from build123d import *

# Parameters (mm, degrees)
BOSS_EXTRUDE1_DEPTH = 55
BOSS_EXTRUDE2_DEPTH = 4
CUT_EXTRUDE1_DEPTH  = 4
SKETCH6_R           = 7
BOSS_EXTRUDE3_DEPTH = 2
SKETCH7_R           = 6
CUT_EXTRUDE2_DEPTH  = 2
SKETCH8_R           = 1.613905717
CUT_EXTRUDE4_DEPTH  = 13
SKETCH9_R           = 6
CUT_EXTRUDE5_DEPTH  = 2
SKETCH11_R          = 1.615
CUT_EXTRUDE6_DEPTH  = 6
FILLET1_R           = 2
SKETCH14_R          = 7
SKETCH14_R_2        = 6
BOSS_EXTRUDE5_DEPTH = 2
CUT_EXTRUDE7_START  = -6
SKETCH15_R          = 1.615
SKETCH15_R_2        = 1.613905717
CUT_EXTRUDE7_DEPTH  = 6
SKETCH16_R          = 1
CUT_EXTRUDE9_DEPTH  = 6
CUT_EXTRUDE10_START = -6
SKETCH17_R          = 1
CUT_EXTRUDE10_DEPTH = 6
SKETCH18_W          = 2.103885612
SKETCH18_H          = 10
CUT_EXTRUDE12_DEPTH = 3
CUT_EXTRUDE13_REACH = 90.057
SKETCH19_R          = 0.8


with BuildPart() as part:
    # Sketch1 → Boss-Extrude1 (new body)
    with BuildSketch(Plane(origin=(0, 0, 0), x_dir=(1, 0, 0), z_dir=(0, 1, 0))):
        with BuildLine():
            Line((-43, 25), (43, 25))
            ThreePointArc((43, 25), (44.414213562, 24.414213562), (45, 23))
            Line((45, 23), (45, -23))
            ThreePointArc((45, -23), (44.414213562, -24.414213562), (43, -25))
            Line((43, -25), (-43, -25))
            ThreePointArc((-43, -25), (-44.414213562, -24.414213562), (-45, -23))
            Line((-45, -23), (-45, 23))
            ThreePointArc((-45, 23), (-44.414213562, 24.414213562), (-43, 25))
        make_face()
        with BuildLine():
            Line((-5, 18), (-5, -18))
            ThreePointArc((-5, -18), (-5.878679656, -20.121320344), (-8, -21))
            Line((-8, -21), (-39, -21))
            ThreePointArc((-39, -21), (-40.414213562, -20.414213562), (-41, -19))
            Line((-41, -19), (-41, 19))
            ThreePointArc((-41, 19), (-40.414213562, 20.414213562), (-39, 21))
            Line((-39, 21), (-8, 21))
            ThreePointArc((-8, 21), (-5.878679656, 20.121320344), (-5, 18))
        make_face(mode=Mode.SUBTRACT)
        with BuildLine():
            Line((41, 19), (41, -18))
            ThreePointArc((41, -18), (40.121320344, -20.121320344), (38, -21))
            Line((38, -21), (8, -21))
            ThreePointArc((8, -21), (5.878679656, -20.121320344), (5, -18))
            Line((5, -18), (5, 18))
            ThreePointArc((5, 18), (5.878679656, 20.121320344), (8, 21))
            Line((8, 21), (39, 21))
            ThreePointArc((39, 21), (40.414213562, 20.414213562), (41, 19))
        make_face(mode=Mode.SUBTRACT)
    extrude(amount=BOSS_EXTRUDE1_DEPTH)

    # Sketch2 → Boss-Extrude2 (add)
    with BuildSketch(Plane.XZ):
        with BuildLine():
            Line((45, 23), (45, -23))
            ThreePointArc((45, -23), (44.414213562, -24.414213562), (43, -25))
            Line((43, -25), (-43, -25))
            ThreePointArc((-43, -25), (-44.414213562, -24.414213562), (-45, -23))
            Line((-45, -23), (-45, 23))
            ThreePointArc((-45, 23), (-44.414213562, 24.414213562), (-43, 25))
            Line((-43, 25), (43, 25))
            ThreePointArc((43, 25), (44.414213562, 24.414213562), (45, 23))
        make_face()
    extrude(amount=-BOSS_EXTRUDE2_DEPTH)

    # Sketch5 → Cut-Extrude1 (cut)
    with BuildSketch(Plane(origin=(0, 55, 0), x_dir=(1, 0, 0), z_dir=(0, 1, 0))):
        with BuildLine():
            Line((-40, 23), (40, 23))
            ThreePointArc((40, 23), (42.121320344, 22.121320344), (43, 20))
            Line((43, 20), (43, -20))
            ThreePointArc((43, -20), (42.121320344, -22.121320344), (40, -23))
            Line((40, -23), (-40, -23))
            ThreePointArc((-40, -23), (-42.121320344, -22.121320344), (-43, -20))
            Line((-43, -20), (-43, 20))
            ThreePointArc((-43, 20), (-42.121320344, 22.121320344), (-40, 23))
        make_face()
    extrude(amount=-CUT_EXTRUDE1_DEPTH, mode=Mode.SUBTRACT)

    # Sketch6 → Boss-Extrude3 (add)
    with BuildSketch(Plane.XY.offset(25)):
        with Locations(Location((-25, 20, 0), (0, 0, 180))):
            Circle(SKETCH6_R)
        with Locations(Location((25, 20, 0), (0, 0, 180))):
            Circle(SKETCH6_R)
    extrude(amount=BOSS_EXTRUDE3_DEPTH)

    # Sketch7 → Cut-Extrude2 (cut)
    with BuildSketch(Plane.XY.offset(27)):
        with Locations((25, 20)):
            Circle(SKETCH7_R)
    extrude(amount=-CUT_EXTRUDE2_DEPTH, mode=Mode.SUBTRACT)

    # Sketch8 → Cut-Extrude4 (cut)
    with BuildSketch(Plane.XY.offset(25)):
        with Locations((25, 20)):
            Circle(SKETCH8_R)
    extrude(amount=-CUT_EXTRUDE4_DEPTH, mode=Mode.SUBTRACT)

    # Sketch9 → Cut-Extrude5 (cut)
    with BuildSketch(Plane.XY.offset(27)):
        with Locations((-25, 20)):
            Circle(SKETCH9_R)
    extrude(amount=-CUT_EXTRUDE5_DEPTH, mode=Mode.SUBTRACT)

    # Sketch11 → Cut-Extrude6 (cut)
    with BuildSketch(Plane.XY.offset(25)):
        with Locations((-25, 20)):
            Circle(SKETCH11_R)
    extrude(amount=-CUT_EXTRUDE6_DEPTH, mode=Mode.SUBTRACT)

    # Fillet1
    fillet1_edges = [part.edges().sort_by_distance(p)[0] for p in [
        (0, 0, -25),
        (44.414213562, 0, -24.414213562),
        (45, 0, 0),
        (44.414213562, 0, 24.414213562),
        (0, 0, 25),
        (-44.414213562, 0, 24.414213562),
        (-45, 0, 0),
        (-44.414213562, 0, -24.414213562),
    ]]
    fillet(fillet1_edges, radius=FILLET1_R)

    # Sketch14 → Boss-Extrude5 (add)
    # profile 1 of 2: a face of its own
    with BuildSketch(Plane(origin=(0, 0, -25), x_dir=(-1, 0, 0), z_dir=(0, 0, -1))):
        with Locations((-25, 20)):
            Circle(SKETCH14_R)
        with Locations(Location((-25, 20, 0), (0, 0, 180))):
            Circle(SKETCH14_R_2, mode=Mode.SUBTRACT)
    # profile 2 of 2: a face of its own
    with BuildSketch(Plane(origin=(0, 0, -25), x_dir=(-1, 0, 0), z_dir=(0, 0, -1))):
        with Locations((25, 20)):
            Circle(SKETCH14_R)
        with Locations(Location((25, 20, 0), (0, 0, 180))):
            Circle(SKETCH14_R_2, mode=Mode.SUBTRACT)
    extrude(amount=BOSS_EXTRUDE5_DEPTH)

    # Sketch15 → Cut-Extrude7 (cut)
    with BuildSketch(Plane(origin=(0, 0, -25), x_dir=(-1, 0, 0), z_dir=(0, 0, -1)).offset(CUT_EXTRUDE7_START)):
        with Locations(Location((25, 20, 0), (0, 0, 180))):
            Circle(SKETCH15_R)
        with Locations(Location((-25, 20, 0), (0, 0, 180))):
            Circle(SKETCH15_R_2)
    extrude(amount=CUT_EXTRUDE7_DEPTH, mode=Mode.SUBTRACT)

    # Sketch16 → Cut-Extrude9 (cut)
    with BuildSketch(Plane(origin=(45, 0, 0), x_dir=(0, 0, -1), z_dir=(1, 0, 0))):
        with Locations((-2.5, 13)):
            Circle(SKETCH16_R)
        with Locations(Location((2.5, 13, 0), (0, 0, 180))):
            Circle(SKETCH16_R)
    extrude(amount=-CUT_EXTRUDE9_DEPTH, mode=Mode.SUBTRACT)

    # Sketch17 → Cut-Extrude10 (cut)
    with BuildSketch(Plane.ZY.offset(45).offset(CUT_EXTRUDE10_START)):
        with Locations((-2.5, 13)):
            Circle(SKETCH17_R)
        with Locations(Location((2.5, 13, 0), (0, 0, 180))):
            Circle(SKETCH17_R)
    extrude(amount=CUT_EXTRUDE10_DEPTH, mode=Mode.SUBTRACT)

    # Sketch18 → Cut-Extrude12 (cut)
    with BuildSketch(Plane(origin=(0, 55, 0), x_dir=(1, 0, 0), z_dir=(0, 1, 0))):
        with Locations((43.955041237, 0)):
            Rectangle(SKETCH18_W, SKETCH18_H)
        with Locations((-43.955041237, 0)):
            Rectangle(SKETCH18_W, SKETCH18_H)
    extrude(amount=-CUT_EXTRUDE12_DEPTH, mode=Mode.SUBTRACT)

    # Cut-Extrude13: up to this face of the body (flat: up to its plane)
    cut_extrude13_end = Plane(part.part.faces().sort_by_distance((0, 29.115734207, -25))[0])
    # Sketch19 → Cut-Extrude13 (cut, up to the picked face)
    with BuildSketch(Plane.XY.offset(25), mode=Mode.PRIVATE) as cut_extrude13_sk1:
        with Locations((-3, 53)):
            Circle(SKETCH19_R)
    cut_extrude13_tool1 = split(extrude(cut_extrude13_sk1.sketch, amount=-CUT_EXTRUDE13_REACH, mode=Mode.PRIVATE), bisect_by=cut_extrude13_end, keep=Keep.BOTH, mode=Mode.PRIVATE)
    # Sketch19 → Cut-Extrude13 (cut, up to the picked face)
    with BuildSketch(Plane.XY.offset(25), mode=Mode.PRIVATE) as cut_extrude13_sk2:
        with Locations((3, 53)):
            Circle(SKETCH19_R)
    cut_extrude13_tool2 = split(extrude(cut_extrude13_sk2.sketch, amount=-CUT_EXTRUDE13_REACH, mode=Mode.PRIVATE), bisect_by=cut_extrude13_end, keep=Keep.BOTH, mode=Mode.PRIVATE)
    add(cut_extrude13_tool1.solids().sort_by(Axis((-3, 53, 25), (0, 0, -1)))[0], mode=Mode.SUBTRACT)
    add(cut_extrude13_tool2.solids().sort_by(Axis((3, 53, 25), (0, 0, -1)))[0], mode=Mode.SUBTRACT)


solid = part.part
Build history of the part. All positions in model axes, mm. A direction names the side the tool comes from. Round coordinates to 2 decimals unless told otherwise and drop trailing zeros. Write each loop counter-clockwise with the first axis right and the second up, starting at its lowest first coordinate (ties: lowest second). Pieces come first, ordered by that corner, then holes. Notation, with made-up numbers: (22.25, -2.75) - (66.25, -2.75) arc R37 ccw to (66.25, 35.25) - close; hole circle Ø11 at (66.5, -10.5). An arc over 180 degrees is marked (long way). Use CSV: the item, a comma, the result in double quotes.
(1) Wall check: line 1 (X direction, y = 43, z = -10); line 2 (Z direction, x = 27.5, y = 47); line 3 (X direction, y = 52, z = -16.5). Give the ranges that are in metal, low to high.
Response:
line 1,"-45 to -41, -5 to 5, 41 to 45"
line 2,"-25 to -21, 21 to 25"
line 3,"-45 to -43, 43 to 45"
(2) 3-axis set-ups, long thin cutter, end or side, ignore diameter. For faces 1 (the cylindrical face through (-5.86, 27.17, 20.1)), 2 (the cylindrical face through (20.58, 15.94, -25.99)), 3 (the cylindrical face through (43.028, 12.024, 2.717)), 4 (the cylindrical face through (23.72, 20.98, -22.97)), 5 (the flat face through (-44, 52, 0)): which of +Z, -Z, +X, -X, +Y, -Y reach the whole face in a straight line?
Response:
face 1,"+Y"
face 2,"-Z"
face 3,"+X"
face 4,"+Z, -Z"
face 5,"+X, -X, +Y"
(3) Mould opens along Z. For faces 6 (the cylindrical face through (-42.972, 12.024, -2.717)), 7 (the cylindrical face through (-19.445, 24.259, 25.986)), 8 (the cylindrical face through (40.4, 27.17, -20.43)) say: pulls with the +Z half, pulls with the -Z half, needs draft (parallel to the pull), parting line crosses it, or undercut.
Response:
face 6,"undercut"
face 7,"needs draft"
face 8,"undercut"
(4) Pin check, flat tips, straight feed: P1, Ø3.5, axis at x = -24.5, y = 21.5, coming from the -Z side; P2, Ø4, axis at x = -25, y = 20, coming from the +Z side; P3, Ø14, axis at x = 14.5, z = 5.5, coming from the +Y side. Stop position of each tip, or through.
Response:
P1,"z = -25"
P2,"z = 25"
P3,"y = 4"
(5) Band-saw the part on A-A (y = 28). Write the cut outline in (x, z).
Response:
outline,"(-45, -23) arc R2 ccw to (-43, -25) - (43, -25) arc R2 ccw to (45, -23) - (45, 23) arc R2 ccw to (43, 25) - (-43, 25) arc R2 ccw to (-45, 23) - close; hole (-41, -19) arc R2 ccw to (-39, -21) - (-8, -21) arc R3 ccw to (-5, -18) - (-5, 18) arc R3 ccw to (-8, 21) - (-39, 21) arc R2 ccw to (-41, 19) - close; hole (5, -18) arc R3 ccw to (8, -21) - (39, -21) arc R2 ccw to (41, -19) - (41, 18) arc R3 ccw to (38, 21) - (8, 21) arc R3 ccw to (5, 18) - close"
(6) Band-saw the part on D-D (z = 15.5). Write the cut outline in (x, y).
Response:
outline,"(-45, 2) arc R2 ccw to (-43, 0) - (43, 0) arc R2 ccw to (45, 2) - (45, 55) - (43, 55) - (43, 51) - (41, 51) - (41, 4) - (5, 4) - (5, 51) - (-5, 51) - (-5, 4) - (-41, 4) - (-41, 51) - (-43, 51) - (-43, 55) - (-45, 55) - close"
(7) Band-saw the part on B-B (x = 35). Write the cut outline in (y, z), plus the area to 3 significant figures.
Response:
outline,"(0, -23) arc R2 ccw to (2, -25) - (55, -25) - (55, -23) - (51, -23) - (51, -21) - (4, -21) - (4, 21) - (51, 21) - (51, 23) - (55, 23) - (55, 25) - (2, 25) arc R2 ccw to (0, 23) - close"
area,"590 mm²"
(8) Band-saw the part on C-C (x = 25). Give the number of separate pieces and of enclosed holes in the cut face, plus the area to 3 significant figures.
Response:
separate pieces,"3"
enclosed holes,"0"
area,"572 mm²"
